Input: part model. Units: mm. Frame: model coordinates. Face numbers are marked on the shaded views. Round coordinates to 2 decimals unless told otherwise and drop trailing zeros. Loops run counter-clockwise (first coordinate to the right, second up) from the corner with the lowest first, then second, coordinate; pieces in that order, holes last. Notation, with made-up numbers: (63, 7.25) -> (112, 7.25) arc R11 ccw to (112, 25.25) -> close; hole circle Ø1 at (38, 1). An arc over 180 degrees is marked (long way). Answer as a JSON object with one key per item and string values. Group by question number.
Item 1: Section query C-C on y = -110. Return loops of the section in (x, z).
Item 2: Section query A-A on x = 0. Return loops of the section in (y, z).
Item 3: Pin query (flat end, axial travel): pin 1 (12 mm diameter, centred on x = 48.5, y = 12, fed in from +Z); pin 2 (3 mm diameter, centred on y = 189, z = 76, fed in from +X); pin 3 (10 mm diameter, centred on y = 21, z = 29, fed in from -X). Return the tip coordinate at first contact, or that it passes through.
Item 4: Draft query along Z for the marked faces 1 and 2. Return one class per face: released by +Z, released by -Z, zero draft, split by the parting line, or undercut.
Item 5: Section query B-B on z = 0. Return loops of the section in (x, y).
Item 6: Material intervals for line 1 (Z direction, x = 0, y = 18); line 2 (Z direction, x = -4.5, y = 0); line 3 (X direction, y = -104.5, z = 84.5), sorted ascending. Write a range as [from, to].
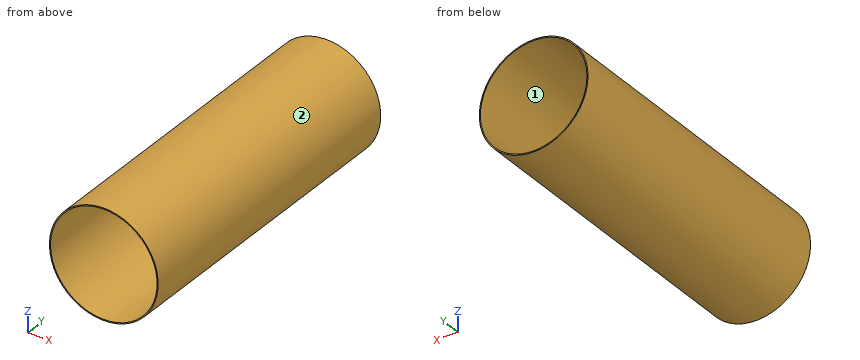
Autodesk Inventor part; units mm, degrees
ref_plane "YZ Plane" through (0, 0, 0) normal (1, 0, 0) x (0, 1, 0)
ref_plane "XZ Plane" through (0, 0, 0) normal (0, 1, 0) x (-1, 0, 0)
ref_plane "XY Plane" through (0, 0, 0) normal (0, 0, 1) x (1, 0, 0)
sketch "Szkic8" plane through (0, 0, 0) normal (0, 1, 0) x (-1, 0, 0)
  circle A0 centre (0, 0) radius 102
  circle A1 centre (0, 0) radius 100
  dimension "d53" = 204
  dimension "d54" = 2
extrude "Wyciągnięcie proste2" add sketch "Szkic8" along normal mid plane 600
sketch "Szkic13" plane through (0, 0, 0) normal (0, 0, 1) x (1, 0, 0)
  circle A0 centre (0, 0) radius 52
  circle A1 centre (0, 0) radius 50
  dimension "d67" = 104
  dimension "d68" = 2
extrude "Wyciągnięcie proste6" add sketch "Szkic13" along normal blind 55.5
sketch "Szkic14" plane through (0, 0, 55.5) normal (0, 0, 1) x (1, 0, 0)
  circle A0 centre (0, 0) radius 50
extrude "Wyciągnięcie proste7" cut sketch "Szkic14" against normal blind 55.5
sketch "Szkic15" plane through (0, -300, 0) normal (0, -1, 0) x (1, 0, 0)
  circle A0 centre (0, 0) radius 100
extrude "Wyciągnięcie proste8" cut sketch "Szkic15" against normal blind 600
fillet "Zaokrąglenie3" [suppressed]
fillet "Zaokrąglenie4" [suppressed]
equation "\"d53\" = OD"
equation "\"d54\" = THK"
equation "\"d55\" = L1"
equation "\"d67\" = OD2"
equation "\"d68\" = THK"
equation "\"d69\" = L2"
equation "\"d71\" = L2"
equation "\"d73\" = L1"
equation "\"d75\" = THK"
equation "\"d76\" = 2 * THK"
equation "\"SzerokośćGięciaPodcięcia\" = Grubość"
equation "\"RozmiarPodcięciaNarożnika\" = 4 * Grubość"
equation "\"PromieńPrzejścia\" = PromieńGięcia"
equation "\"Rozmiar_promienia_Jacobiego\" = PromieńGięcia"
equation "\"Wielk_odstępu\" = Grubość"
equation "\"d2\" = PromieńGięcia"
equation "\"d23\" = PromieńGięcia"
equation "\"OD\" = 204"
equation "\"THK\" = 2"
equation "\"L1\" = 600"
equation "\"L2\" = 55.5"
equation "\"OD2\" = 104"
properties part number "Trójnik red. krótki  Ø204 104 204 s=2 L=600" material "304"
Solved:
{
 "1": {"outline": "circle Ø204 at (0, 0); hole circle Ø200 at (0, 0)"},
 "2": {"outline": "(-300, -102) -> (300, -102) -> (300, -100) -> (-300, -100) -> close; (-300, 100) -> (300, 100) -> (300, 102) -> (-300, 102) -> close"},
 "3": {"pin 1": "z = 92.72", "pin 2": "x = 69.67", "pin 3": "x = -99.14"},
 "4": {"face 1": "undercut", "face 2": "split by the parting line"},
 "5": {"outline": "(-102, -300) -> (-100, -300) -> (-100, 300) -> (-102, 300) -> close; (100, -300) -> (102, -300) -> (102, 300) -> (100, 300) -> close"},
 "6": {"line 1": "[-102, -100], [100, 102]", "line 2": "[-101.9, -99.9], [99.9, 101.9]", "line 3": "[-57.13, -53.48], [53.48, 57.13]"}
}
